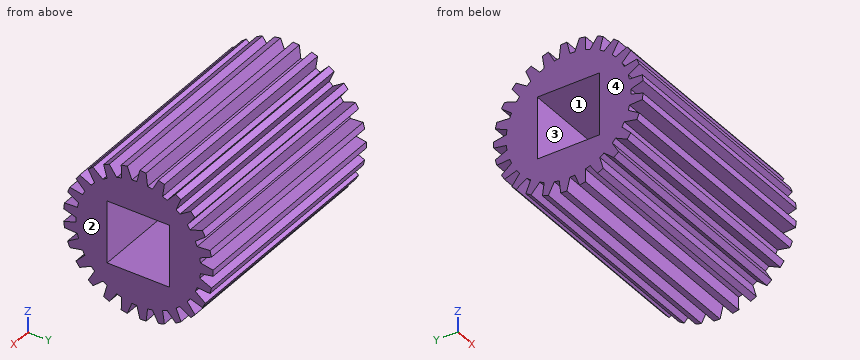
```python
from build123d import *

# Parameters (mm, degrees)
BOSS_EXTRUDE2_START      = -13
BOSS_EXTRUDE2_DEPTH      = 18
BOSS_EXTRUDE3_DEPTH      = 5
BOSS_EXTRUDE3_DEPTH_BACK = 13
SKETCH3_R                = 5
CIRPATTERN1_COUNT        = 25
SKETCH4_W                = 5
SKETCH4_H                = 5
CUT_EXTRUDE1_DEPTH       = 18


with BuildPart() as part:
    # Sketch2 → Boss-Extrude2 (new body)
    with BuildSketch(Plane(origin=(0, 0, 0), x_dir=(0, 0, -1), z_dir=(1, 0, 0)).offset(BOSS_EXTRUDE2_START)):
        with BuildLine():
            ThreePointArc((0.429587035, 4.981511315), (0, 5), (-0.429587035, 4.981511315))
            Line((-0.429587035, 4.981511315), (-0.700772987, 3.443539352))
            Line((-0.700772987, 3.443539352), (0.700772987, 3.443539352))
            Line((0.700772987, 3.443539352), (0.429587035, 4.981511315))
        make_face()
        with BuildLine():
            Line((0.25, 6), (-0.25, 6))
            Line((-0.25, 6), (-0.429587035, 4.981511315))
            ThreePointArc((-0.429587035, 4.981511315), (0, 5), (0.429587035, 4.981511315))
            Line((0.429587035, 4.981511315), (0.25, 6))
        make_face()
    boss_extrude2 = extrude(amount=BOSS_EXTRUDE2_DEPTH)

    # Sketch3 → Boss-Extrude3 (add, two sides: drawn at the far end of the back side and taken through both)
    with BuildSketch(Plane(origin=(0, 0, 0), x_dir=(0, 0, -1), z_dir=(1, 0, 0)).offset(-BOSS_EXTRUDE3_DEPTH_BACK)):
        Circle(SKETCH3_R)
    extrude(amount=BOSS_EXTRUDE3_DEPTH + BOSS_EXTRUDE3_DEPTH_BACK)

    # CirPattern1: Boss-Extrude2 ×25 about axis
    cirpattern1_axis = Axis((0, 0, 0), (1, 0, 0))
    for i in range(1, CIRPATTERN1_COUNT):
        add(boss_extrude2.rotate(cirpattern1_axis, i * 360 / CIRPATTERN1_COUNT))

    # Sketch4 → Cut-Extrude1 (cut)
    with BuildSketch(Plane(origin=(5, 0, 0), x_dir=(0, 0, -1), z_dir=(1, 0, 0))):
        Rectangle(SKETCH4_W, SKETCH4_H)
    extrude(amount=-CUT_EXTRUDE1_DEPTH, mode=Mode.SUBTRACT)


solid = part.part
```
Geometry: final body of the model. Coordinates: model frame, mm. Face numbers are marked on the shaded views. A direction names the side the tool comes from. Coordinates: 2 decimals unless noted, no trailing zeros. Write each question's results on one line, items separated by ' | '.
(1) Line query: line 1 (Z direction, x = -12, y = -4.5); line 2 (Y direction, x = -10.5, z = -5.25); line 3 (Z direction, x = -1.25, y = 4). Output: solid intervals per line, ascending. Write a range as [from, to].
Values found:
line 1: z = [-3.63, -2.81], [-2.24, 2.24], [2.81, 3.63] | line 2: y = [-2.76, -2.13], [-1.36, -0.62], [-0.06, 0.71], [1.33, 2.04] | line 3: z = [-4.16, -3.2], [-3, 3], [3.2, 4.16]
(2) Set-up query: the marked faces 1 and 2. Return all of +Z, -Z, +X, -X, +Y, -Y with unobstructed straight access to the full face (end or side cutting, diameter ignored); none if empty.
Values found:
face 1: +X, -X | face 2: +Z, -Z, +X, +Y, -Y
(3) First-contact query: pin 1 Ø3 at (x, z) = (-9.5, 4.5) entering from +Y; pin 2 Ø6 at (x, y) = (-8, 2) entering from +Z; pin 3 Ø1.5 at (x, y) = (-10, 1.5) entering from -Z. Flat tips, straight axial feed; report the tip coordinate or a pass-through.
Values found:
pin 1: stops at y = 5.2 | pin 2: stops at z = 6 | pin 3: stops at z = -5.78
(4) Mould query, pull axis Z, two halves, no side actions, for the marked faces 3 and 4. Classes: +Z half, -Z half, draft (parallel to the pull), parting line (faces both ways), or undercut.
Values found:
face 3: undercut | face 4: draft
